```python
from build123d import *

# Parameters (mm, degrees)
SKETCH1_W           = 203
SKETCH1_H           = 280
BOSS_EXTRUDE1_DEPTH = 6.35
SKETCH2_R           = 1.475
CUT_EXTRUDE1_DEPTH  = 6.35
SKETCH3_W           = 6.35
SKETCH3_H           = 12
SKETCH3_W_2         = 16
SKETCH3_H_2         = 25
CUT_EXTRUDE2_DEPTH  = 6.35
FILLET1_R           = 60


with BuildPart() as part:
    # Sketch1 → Boss-Extrude1 (new body)
    with BuildSketch(Plane.XY):
        Rectangle(SKETCH1_W, SKETCH1_H)
    extrude(amount=BOSS_EXTRUDE1_DEPTH)

    # Sketch2 → Cut-Extrude1 (cut)
    with BuildSketch(Plane.XY.offset(6.35)):
        with Locations((60.26, 95.875)):
            Circle(SKETCH2_R)
        with Locations((75.5, 95.875)):
            Circle(SKETCH2_R)
        with Locations((60.26, 64.125)):
            Circle(SKETCH2_R)
        with Locations((75.5, 64.125)):
            Circle(SKETCH2_R)
        with Locations((-75.5, 64.125)):
            Circle(SKETCH2_R)
        with Locations((-60.26, 64.125)):
            Circle(SKETCH2_R)
        with Locations((-75.5, 95.875)):
            Circle(SKETCH2_R)
        with Locations((-60.26, 95.875)):
            Circle(SKETCH2_R)
    extrude(amount=-CUT_EXTRUDE1_DEPTH, mode=Mode.SUBTRACT)

    # Sketch3 → Cut-Extrude2 (cut)
    with BuildSketch(Plane.XY.offset(6.35)):
        with Locations((-22, -131)):
            Rectangle(SKETCH3_W, SKETCH3_H)
        with Locations((-22, -107)):
            Rectangle(SKETCH3_W, SKETCH3_H)
        with Locations((-22, -83)):
            Rectangle(SKETCH3_W, SKETCH3_H)
        with Locations((2, -127.5)):
            Rectangle(SKETCH3_W_2, SKETCH3_H_2)
    extrude(amount=-CUT_EXTRUDE2_DEPTH, mode=Mode.SUBTRACT)

    # Fillet1
    fillet1_edges = [part.edges().sort_by_distance(p)[0] for p in [
        (101.5, -140, 3.175),
        (-101.5, -140, 3.175),
    ]]
    fillet(fillet1_edges, radius=FILLET1_R)


solid = part.part
```
For this review, take the finished solid that the model builds, in its own axes (mm). A direction names the side the tool comes from. Coordinates: 2 decimals unless noted, no trailing zeros. Order: outer loops, then holes, each group sorted by start corner. A loop starts at its lowest first (then second) coordinate and runs counter-clockwise, first axis right, second up. Notation, with made-up numbers: (82.25, -36) -> (128.25, -36) arc R15 ccw to (128.25, -30) -> close; hole circle Ø7 at (12, 42.25). An arc over 180 degrees is marked (long way). Use CSV: the item, a comma, the result in double quotes. Start each with the question number.
Item 1: For faces 1 (the face through (-24, -140, 3)), 2 (the face through (-22, -125, 3)), 3 (the face through (-6, -128, 3)), list the 3-axis set-ups (+Z, -Z, +X, -X, +Y, -Y) from which the entire face can be reached by the end or side of a thin tool; tool diameter is ignored.
Item 2: Draft analysis for pull direction X (two halves, no side actions). For faces 4 (the face through (101.5, 28, 3)), 5 (the face through (-1, 2, 6.35)), 6 (the face through (-25.175, -107, 3)), state which applies: pulls with the +X half, pulls with the -X half, needs draft (parallel to the pull), parting line crosses it, or undercut.
Item 3: We need section D-D, the plane x = -89. Give the boundary of the cut face in (y, z), then the cut area to 3 significant figures.
Item 4: We need section B-B, the plane z = 2.75. Give the number of separate pieces and of enclosed holes in the cut face, then the cut area to 3 significant figures.
Item 5: We need section C-C, the plane x = 87. Give the boundary of the cut face in (y, z), then the cut area to 3 significant figures.
Item 6: We need section A-A, the plane y = -86. Give the boundary of the cut face in (x, z) (3 decimals), then the cut area to 3 significant figures.
Item 7: Insertion check: pin 1 (2.5 mm diameter, centred on x = -75.5, y = 95.875, fed in from +Z); pin 2 (1 mm diameter, centred on x = -46, y = -46, fed in from -Z). Each pin has a flat end and moves straight along its axis. Give the tip position at first contact, or say it passes through.
Item 8: Wall thickness on probe 1 along Y at (x, z) = (-60.26, 2.75); probe 2 along Y at (x, z) = (-60, 1); probe 3 along X at (y, z) = (65, 2.5): over which ranges is each line inside the solid? List them lowest first.
Derived:
1,face 1,"+Z, -Z, +X, -X, -Y"
1,face 2,"+Z, -Z"
1,face 3,"+Z, -Z, -Y"
2,face 4,"pulls with the +X half"
2,face 5,"needs draft"
2,face 6,"undercut"
3,outline,"(-116.66, 0) -> (140, 0) -> (140, 6.35) -> (-116.66, 6.35) -> close"
3,area,"1,630 mm^2"
4,separate pieces,"1"
4,enclosed holes,"11"
4,area,"54,600 mm^2"
5,outline,"(-119.11, 0) -> (140, 0) -> (140, 6.35) -> (-119.11, 6.35) -> close"
5,area,"1,650 mm^2"
6,outline,"(-101.199, 0) -> (-25.175, 0) -> (-25.175, 6.35) -> (-101.199, 6.35) -> close; (-18.825, 0) -> (101.199, 0) -> (101.199, 6.35) -> (-18.825, 6.35) -> close"
6,area,"1,240 mm^2"
7,pin 1,"passes through"
7,pin 2,"stops at z = 0"
8,probe 1,"y = -136.99 to 62.65, 65.6 to 94.4, 97.35 to 140"
8,probe 2,"y = -137.08 to 62.67, 65.58 to 94.42, 97.33 to 140"
8,probe 3,"x = -101.5 to -76.69, -74.31 to -61.45, -59.07 to 59.07, 61.45 to 74.31, 76.69 to 101.5"
